```python
from build123d import *

# Parameters (mm, degrees)
F0_R     = 12.7
F1_DEPTH = 38.1
F2_R     = 6.35
F3_DEPTH = 12.701


with BuildPart() as f1:
    # F0 (on Front) → F1 (new body)
    with BuildSketch(Plane.XZ):
        with BuildLine():
            Line((-33.163997, 19.499587), (-64.999874, 19.499587))
            Line((-64.999874, 19.499587), (-64.999874, 6.799587))
            Line((-64.999874, 6.799587), (62.000126, 6.799587))
            Line((62.000126, 6.799587), (62.000126, 19.499587))
            Line((62.000126, 19.499587), (30.164248, 19.499587))
            ThreePointArc((30.164248, 19.499587), (21.597672, 22.823886), (17.515798, 31.056474))
            ThreePointArc((17.515798, 31.056474), (17.464248, 32.199587), (17.515798, 33.3427))
            ThreePointArc((17.515798, 33.3427), (-1.499874, 51.249587), (-20.515546, 33.3427))
            ThreePointArc((-20.515546, 33.3427), (-20.463997, 32.199587), (-20.515546, 31.056474))
            ThreePointArc((-20.515546, 31.056474), (-24.59742, 22.823886), (-33.163997, 19.499587))
        make_face()
        with Locations((-1.499874, 32.199587)):
            Circle(F0_R, mode=Mode.SUBTRACT)
        with BuildLine():
            ThreePointArc((-20.515546, 33.3427), (-20.549874, 32.199587), (-20.515546, 31.056474))
            ThreePointArc((-20.515546, 31.056474), (-20.463997, 32.199587), (-20.515546, 33.3427))
        make_face()
        with BuildLine():
            ThreePointArc((17.515798, 31.056474), (17.550126, 32.199587), (17.515798, 33.3427))
            ThreePointArc((17.515798, 33.3427), (17.464248, 32.199587), (17.515798, 31.056474))
        make_face()
    extrude(amount=F1_DEPTH)

    # F2 (on face) → F3 (cut, through all)
    with BuildSketch(Plane.XY.offset(19.499587)):
        with Locations((42.950126, -19.05)):
            Circle(F2_R)
        with Locations((-45.949874, -19.05)):
            Circle(F2_R)
    extrude(amount=-F3_DEPTH, mode=Mode.SUBTRACT)


solid = f1.part
```
Design review of the part built by this model. Coordinates are the model's own, in mm. A direction names the side the tool comes from. Give positions to 0.01 mm unless a question says otherwise; leave off trailing zeros. Write each loop counter-clockwise with the first axis right and the second up, starting at its lowest first coordinate (ties: lowest second). Pieces come first, ordered by that corner, then holes. Notation, with made-up numbers: (37.25, 86.25) -> (94.25, 86.25) arc R18 cw to (94.25, 113.25) -> close; hole circle Ø10 at (-16, -40). An arc over 180 degrees is marked (long way). Answer in a Markdown table with one row per item.
(1) Consider section C-C (z = 29.5). State the section outline as (x, y) points.
Results:
| item | result |
|---|---|
| outline | (-20.75, -38.1) -> (-13.91, -38.1) -> (-13.91, 0) -> (-20.75, 0) -> close; (10.91, -38.1) -> (17.75, -38.1) -> (17.75, 0) -> (10.91, 0) -> close |
(2) To check wall thickness, follow probe 1 along X at (y, z) = (-19, 15); probe 2 along X at (y, z) = (-3.5, 31.5); probe 3 along X at (y, z) = (-20.5, 12.5). State the ranges of each line that lie inside material, in increasing order.
Results:
| item | result |
|---|---|
| probe 1 | -65 to -52.3, -39.6 to 36.6, 49.3 to 62 |
| probe 2 | -20.54 to -14.18, 11.18 to 17.54 |
| probe 3 | -65 to -52.13, -39.77 to 36.77, 49.13 to 62 |
(3) Consider section B-B (x = 0). State the section outline as (y, z) points.
Results:
| item | result |
|---|---|
| outline | (-38.1, 6.8) -> (0, 6.8) -> (0, 19.59) -> (-38.1, 19.59) -> close; (-38.1, 44.81) -> (0, 44.81) -> (0, 51.19) -> (-38.1, 51.19) -> close |
(4) For faces 1 (the flat face through (-52, -23, 19.5)), 2 (the flat face through (-2, 0, 19)), 3 (the flat face through (50, -19, 19.5)), list the 3-axis set-ups (+Z, -Z, +X, -X, +Y, -Y) from which the entire face can be reached by the end or side of a thin tool; tool diameter is ignored.
Results:
| item | result |
|---|---|
| face 1 | +Z, -X, +Y, -Y |
| face 2 | +Z, -Z, +X, -X, +Y |
| face 3 | +Z, +X, +Y, -Y |
(5) Clearance check with flat-ended pins moving along their axes: pin 1 (12 mm diameter, centred on y = -12.5, z = 31, fed in from +X); pin 2 (1.5 mm diameter, centred on y = -4, z = 34, fed in from +X); pin 3 (2 mm diameter, centred on y = -27, z = 26.5, fed in from -X). State where each tip first meets the part, or that it passes through.
Results:
| item | result |
|---|---|
| pin 1 | x = 19.7 |
| pin 2 | x = 17.52 |
| pin 3 | x = -22.37 |
(6) Consider section A-A (y = -24). State the section outline as (x, z) points, then the cut area to 3 significant figures.
Results:
| item | result |
|---|---|
| outline | (-65, 6.8) -> (-49.93, 6.8) -> (-49.93, 19.5) -> (-65, 19.5) -> close; (-41.97, 6.8) -> (38.97, 6.8) -> (38.97, 19.5) -> (30.16, 19.5) arc R12.7 cw to (17.52, 31.06) arc R19.05 ccw to (17.52, 33.34) arc R19.05 ccw to (-20.52, 33.34) arc R19.05 ccw to (-20.52, 31.06) arc R12.7 cw to (-33.16, 19.5) -> (-41.97, 19.5) -> close; (46.93, 6.8) -> (62, 6.8) -> (62, 19.5) -> (46.93, 19.5) -> close; hole circle Ø25.4 at (-1.5, 32.2) |
| area | 2,030 mm2 |
(7) Mouldability with a two-part tool opening along X and no side actions: class faces 4 (the flat face through (-2, -19, 6.8)), 5 (the cylindrical face through (-40.084, -21.482, 13.238)), 6 (the flat face through (62, -19, 13)) as +X half, -X half, draft (parallel to the pull), parting line (faces both ways), or undercut.
Results:
| item | result |
|---|---|
| face 4 | draft |
| face 5 | undercut |
| face 6 | +X half |
(8) Consider section D-D (z = 11.5). State the section outline as (x, y) points.
Results:
| item | result |
|---|---|
| outline | (-65, -38.1) -> (62, -38.1) -> (62, 0) -> (-65, 0) -> close; hole circle Ø12.7 at (-45.95, -19.05); hole circle Ø12.7 at (42.95, -19.05) |
